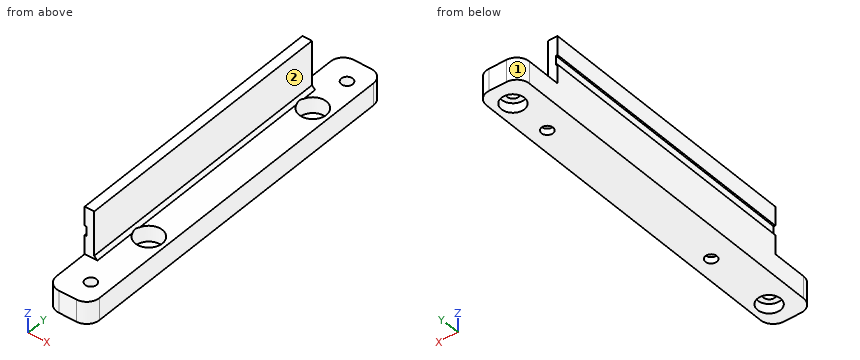
from build123d import *

# Parameters (mm, degrees)
SKETCH008_W     = 13.5
SKETCH008_H     = 115
PAD001_DEPTH    = 22
SKETCH009_W     = 16
SKETCH009_H     = 16
POCKET007_DEPTH = 30
SKETCH010_R     = 1.8
POCKET008_DEPTH = 22.001
SKETCH011_R     = 3.6
POCKET009_DEPTH = 18
SKETCH012_W     = 11
SKETCH012_H     = 85
POCKET010_DEPTH = 15
CHAMFER001_SIZE = 1
SKETCH013_W     = 87.5
SKETCH013_H     = 3
POCKET011_DEPTH = 0.5
SKETCH014_R     = 1.8
POCKET012_DEPTH = 22.001
SKETCH015_R     = 3.6
POCKET013_DEPTH = 3
FILLET003_R     = 4
SKETCH016_R     = 4.25
POCKET014_DEPTH = 5
SKETCH017_R     = 1.8
POCKET015_DEPTH = 19.001


with BuildPart() as part:
    # Sketch008 → Pad001 (new body)
    with BuildSketch(Plane.XY):
        with Locations((-71.25, 57.5)):
            Rectangle(SKETCH008_W, SKETCH008_H)
    extrude(amount=PAD001_DEPTH)

    # Sketch009 → Pocket007 (cut)
    with BuildSketch(Plane(origin=(-78, 0, 0), x_dir=(0, -1, 0), z_dir=(-1, 0, 0))):
        with Locations((-108, 15)):
            Rectangle(SKETCH009_W, SKETCH009_H)
        with Locations((-7, 15)):
            Rectangle(SKETCH009_W, SKETCH009_H)
    extrude(amount=-POCKET007_DEPTH, mode=Mode.SUBTRACT)

    # Sketch010 → Pocket008 (cut, through all)
    with BuildSketch(Plane.XY.offset(22)):
        with Locations((-70.00164, 94.105309)):
            Circle(SKETCH010_R)
        with Locations((-69.993416, 30.102623)):
            Circle(SKETCH010_R)
    extrude(amount=-POCKET008_DEPTH, mode=Mode.SUBTRACT)

    # Sketch011 → Pocket009 (cut)
    with BuildSketch(Plane.XY.offset(22)):
        with Locations((-70, 94.117142)):
            Circle(SKETCH011_R)
        with Locations((-70, 30.122299)):
            Circle(SKETCH011_R)
    extrude(amount=-POCKET009_DEPTH, mode=Mode.SUBTRACT)

    # Sketch012 → Pocket010 (cut)
    with BuildSketch(Plane.XY.offset(22)):
        with Locations((-69.5, 57.5)):
            Rectangle(SKETCH012_W, SKETCH012_H)
    extrude(amount=-POCKET010_DEPTH, mode=Mode.SUBTRACT)

    # Chamfer001
    chamfer001_edges = [part.edges().sort_by_distance(p)[0] for p in [
        (-75, 57.5, 7),
    ]]
    chamfer(chamfer001_edges, length=CHAMFER001_SIZE)

    # Sketch013 → Pocket011 (cut)
    with BuildSketch(Plane(origin=(-78, 0, 0), x_dir=(0, -1, 0), z_dir=(-1, 0, 0))):
        with Locations((-57.75, 14.5)):
            Rectangle(SKETCH013_W, SKETCH013_H)
    extrude(amount=-POCKET011_DEPTH, mode=Mode.SUBTRACT)

    # Sketch014 → Pocket012 (cut, through all)
    with BuildSketch(Plane(origin=(0, 0, 0), x_dir=(1, 0, 0), z_dir=(0, 0, -1))):
        with Locations((-70, -7.5)):
            Circle(SKETCH014_R)
        with Locations((-70, -107.5)):
            Circle(SKETCH014_R)
    extrude(amount=-POCKET012_DEPTH, mode=Mode.SUBTRACT)

    # Sketch015 → Pocket013 (cut)
    with BuildSketch(Plane(origin=(0, 0, 0), x_dir=(1, 0, 0), z_dir=(0, 0, -1))):
        with Locations((-70, -7.5)):
            Circle(SKETCH015_R)
        with Locations((-70, -107.5)):
            Circle(SKETCH015_R)
    extrude(amount=-POCKET013_DEPTH, mode=Mode.SUBTRACT)

    # Fillet003
    fillet003_edges = [part.edges().sort_by_distance(p)[0] for p in [
        (-78, 0, 3.5),
        (-64.5, 0, 3.5),
        (-64.5, 115, 3.5),
        (-78, 115, 3.5),
    ]]
    fillet(fillet003_edges, radius=FILLET003_R)

    # Sketch016 → Pocket014 (cut, symmetric)
    with BuildSketch(Plane.XY.offset(7)):
        with Locations((-70, 94.135872)):
            Circle(SKETCH016_R)
        with Locations((-70, 30.123001)):
            Circle(SKETCH016_R)
    extrude(amount=POCKET014_DEPTH, both=True, mode=Mode.SUBTRACT)

    # Sketch017 → Pocket015 (cut, through all)
    with BuildSketch(Plane(origin=(0, 0, 3), x_dir=(1, 0, 0), z_dir=(0, 0, -1))):
        with Locations((-70, 30.106855)):
            Circle(SKETCH017_R)
        with Locations((-70, 94.115112)):
            Circle(SKETCH017_R)
    extrude(amount=-POCKET015_DEPTH, mode=Mode.SUBTRACT)


solid = part.part
Can you work these out from the model? Positions are in its coordinate system, mm. Face numbers are marked on the shaded views. A direction names the side the tool comes from. Give positions to 0.01 mm unless a question says otherwise; leave off trailing zeros. Loops run counter-clockwise (first coordinate to the right, second up) from the corner with the lowest first, then second, coordinate; pieces in that order, holes last. Notation, with made-up numbers: (23.5, 88.25) - (27.5, 88.25) arc R22 cw to (27.5, 114.25) - close; hole circle Ø6 at (71, 88). An arc over 180 degrees is marked (long way). Answer as a JSON object with one key per item and string values.
Q1. Imagine slicing it at A-A on y = 107.5. Write out the boundary of the cut face in (x, z).
Geometry says:
{"outline": "(-78, 0) - (-73.6, 0) - (-73.6, 3) - (-71.8, 3) - (-71.8, 7) - (-78, 7) - close; (-68.2, 3) - (-66.4, 3) - (-66.4, 0) - (-64.5, 0) - (-64.5, 7) - (-68.2, 7) - close"}
Q2. Imagine slicing it at D-D on z = 4. Write out the boundary of the cut face in (x, y).
Geometry says:
{"outline": "(-78, 4) arc R4 ccw to (-74, 0) - (-68.5, 0) arc R4 ccw to (-64.5, 4) - (-64.5, 111) arc R4 ccw to (-68.5, 115) - (-74, 115) arc R4 ccw to (-78, 111) - close; hole circle Ø8.5 at (-70, 30.12); hole circle Ø8.5 at (-70, 94.14); hole circle Ø3.6 at (-70, 7.5); hole circle Ø3.6 at (-70, 107.5)"}
Q3. If I drill on L1, parallel to Y at x = -70, z = 5.9; L2, parallel to X at y = 7.5, z = 1.9; L3, parallel to Y at x = -72.5, z = 4.5, over which ranges is the centre line in solid material (lowest first)?
Geometry says:
{"L1": "0 to 5.7, 9.3 to 25.87, 34.37 to 89.89, 98.39 to 105.7, 109.3 to 115", "L2": "-78 to -73.6, -66.4 to -64.5", "L3": "0 to 26.69, 33.56 to 90.7, 97.57 to 115"}
Q4. Imagine slicing it at C-C on y = 48. Write out the boundary of the cut face in (x, z), plus the area to 4 significant figures.
Geometry says:
{"outline": "(-78, 0) - (-64.5, 0) - (-64.5, 7) - (-74, 7) - (-75, 8) - (-75, 22) - (-78, 22) - (-78, 16) - (-77.5, 16) - (-77.5, 13) - (-78, 13) - close", "area": "138.5 mm²"}
Q5. Which directions (+Z, -Z, +X, -X, +Y, -Y) give clear straight access to the entire face, cutting with the end or side of a thin tool? Please do the marked faces 1 and 2.
Geometry says:
{"face 1": "+Z, -Z, -X, +Y", "face 2": "+Z, +X, +Y, -Y"}
Q6. Imagine slicing it at B-B on x = -76.5. Write out the boundary of the cut face in (y, z).
Geometry says:
{"outline": "(0.88, 0) - (114.12, 0) - (114.12, 7) - (100, 7) - (100, 22) - (15, 22) - (15, 7) - (0.88, 7) - close"}
Q7. Will these pins go through, and if not, where does the flat tip stop? P1, Ø7, axis at x = -70, y = 94.14, coming from the +Z side; P2, Ø6, axis at x = -70, y = 7.5, coming from the -Z side; P3, Ø6, axis at x = -70, y = 107.5, coming from the +Z side; P4, Ø7, axis at x = -70, y = 30.123, coming from the -Z side.
Geometry says:
{"P1": "z = 2", "P2": "z = 3", "P3": "z = 7", "P4": "z = 0"}
